Read the model definition and answer for the solid it produces. Units are mm, in the model's axes. A direction names the side the tool comes from. Coordinates: 2 decimals unless noted, no trailing zeros. Loops run counter-clockwise (first coordinate to the right, second up) from the corner with the lowest first, then second, coordinate; pieces in that order, holes last.
from build123d import *

# Parameters (mm, degrees)
ESQUISSE2_W             = 66
ESQUISSE2_H             = 24
BOSS_EXTRU_1_DEPTH      = 6
ESQUISSE3_W             = 23
ESQUISSE3_H             = 24
ENL_V_MAT_EXTRU_1_DEPTH = 2
ESQUISSE4_R             = 1.8
ENL_V_MAT_EXTRU_2_DEPTH = 5
ESQUISSE5_R             = 2.75
ENL_V_MAT_EXTRU_3_DEPTH = 7
ESQUISSE6_R             = 5.1
ENL_V_MAT_EXTRU_4_DEPTH = 3
CONG_1_R                = 0.75


with BuildPart() as part:
    # Esquisse2 → Boss.-Extru.1 (new body)
    with BuildSketch(Plane.XY):
        with Locations((33, 12)):
            Rectangle(ESQUISSE2_W, ESQUISSE2_H)
    extrude(amount=BOSS_EXTRU_1_DEPTH)

    # Esquisse3 → Enlèv. mat.-Extru.1 (cut)
    with BuildSketch(Plane.XY.offset(6)):
        with Locations((33, 12)):
            Rectangle(ESQUISSE3_W, ESQUISSE3_H)
    extrude(amount=-ENL_V_MAT_EXTRU_1_DEPTH, mode=Mode.SUBTRACT)

    # Esquisse4 → Enlèv. mat.-Extru.2 (cut, through all)
    with BuildSketch(Plane.XY.offset(4)):
        with Locations((33, 16)):
            Circle(ESQUISSE4_R)
    extrude(amount=-ENL_V_MAT_EXTRU_2_DEPTH, mode=Mode.SUBTRACT)

    # Esquisse5 → Enlèv. mat.-Extru.3 (cut, through all)
    with BuildSketch(Plane(origin=(0, 0, 0), x_dir=(-1, 0, 0), z_dir=(0, 0, -1))):
        with Locations((-59, 6)):
            Circle(ESQUISSE5_R)
        with Locations((-7, 6)):
            Circle(ESQUISSE5_R)
    extrude(amount=-ENL_V_MAT_EXTRU_3_DEPTH, mode=Mode.SUBTRACT)

    # Esquisse6 → Enlèv. mat.-Extru.4 (cut)
    with BuildSketch(Plane(origin=(0, 0, 0), x_dir=(-1, 0, 0), z_dir=(0, 0, -1))):
        with Locations((-59, 6)):
            Circle(ESQUISSE6_R)
        with Locations((-7, 6)):
            Circle(ESQUISSE6_R)
    extrude(amount=-ENL_V_MAT_EXTRU_4_DEPTH, mode=Mode.SUBTRACT)

    # Congé1
    cong_1_edges = [part.edges().sort_by_distance(p)[0] for p in [
        (66, 12, 6),
        (55.25, 24, 6),
        (55.25, 0, 6),
        (10.75, 24, 6),
        (21.5, 12, 6),
        (44.5, 12, 6),
        (61.75, 6, 6),
        (9.75, 6, 6),
        (0, 12, 6),
        (10.75, 0, 6),
        (0, 24, 3),
        (66, 24, 3),
        (66, 0, 3),
        (0, 0, 3),
    ]]
    fillet(cong_1_edges, radius=CONG_1_R)


solid = part.part
Q1. Straight lines are drawn through the part: probe 1 along X at (y, z) = (10.5, 2.6); probe 2 along X at (y, z) = (3.5, 3.4); probe 3 along Y at (x, z) = (59, 2). For each, find the intervals that lie inside material, in ascending order.
Findings below:
probe 1: x = 0 to 4.6, 9.4 to 56.6, 61.4 to 66
probe 2: x = 0 to 5.85, 8.15 to 57.85, 60.15 to 66
probe 3: y = 0 to 0.9, 11.1 to 24
Q2. A cutting plane is placed at A-A (x = 33). Give the vertices of the cut face in (y, z).
Findings below:
outline: (0, 0) - (14.2, 0) - (14.2, 4) - (0, 4) - close; (17.8, 0) - (24, 0) - (24, 4) - (17.8, 4) - close
Q3. Flat-ended cylindrical pins translate along their axes: pin 1 Ø4 at (x, y) = (33, 16) entering from +Z; pin 2 Ø7 at (x, y) = (59, 6) entering from -Z; pin 3 Ø1 at (x, z) = (23, 5) entering from -Y. Find the tip coordinate at first contact, or state that the pin passes through.
Findings below:
pin 1: stops at z = 4
pin 2: stops at z = 3
pin 3: passes through
Q4. A cutting plane is placed at B-B (z = 1.6). Give the vertices of the cut face in (x, y).
Findings below:
outline: (0, 0.75) arc R0.75 ccw to (0.75, 0) - (65.25, 0) arc R0.75 ccw to (66, 0.75) - (66, 23.25) arc R0.75 ccw to (65.25, 24) - (0.75, 24) arc R0.75 ccw to (0, 23.25) - close; hole circle Ø10.2 at (7, 6); hole circle Ø3.6 at (33, 16); hole circle Ø10.2 at (59, 6)
Q5. A cutting plane is placed at D-D (y = 20.75). Give the vertices of the cut face in (x, z).
Findings below:
outline: (0, 0) - (66, 0) - (66, 5.25) arc R0.75 ccw to (65.25, 6) - (45.25, 6) arc R0.75 ccw to (44.5, 5.25) - (44.5, 4) - (21.5, 4) - (21.5, 5.25) arc R0.75 ccw to (20.75, 6) - (0.75, 6) arc R0.75 ccw to (0, 5.25) - close
Q6. A cutting plane is placed at C-C (y = 16). Give the vertices of the cut face in (x, z), then the cut area to 3 significant figures.
Findings below:
outline: (0, 0) - (31.2, 0) - (31.2, 4) - (21.5, 4) - (21.5, 5.25) arc R0.75 ccw to (20.75, 6) - (0.75, 6) arc R0.75 ccw to (0, 5.25) - close; (34.8, 0) - (66, 0) - (66, 5.25) arc R0.75 ccw to (65.25, 6) - (45.25, 6) arc R0.75 ccw to (44.5, 5.25) - (44.5, 4) - (34.8, 4) - close
area: 335 mm2
Q7. Which of the six approach directions +Z, -Z, +X, -X, +Y, -Y give full straight-line access (tool end or side, diameter ignored) to faces 1 (the face through (33, 12, 4)), 2 (the face through (4.8, 3.8, 3)), 3 (the face through (0, 12, 3))?
Findings below:
face 1: +Z, +Y, -Y
face 2: -Z
face 3: +Z, -Z, -X, +Y, -Y
Q8. Determine the mould class of faces 4 (the face through (33, 24, 3)), 5 (the face through (33, 0, 3)), 6 (the face through (21.5, 12, 5)), 7 (the face through (4.26, 10.3, 1.48)) for opening direction Y: +Y half, -Y half, draft (parallel to the pull), parting line (faces both ways), or undercut.
Findings below:
face 4: +Y half
face 5: -Y half
face 6: draft
face 7: undercut
